```python
from build123d import *

# Parameters (mm, degrees)
F0_R     = 1.27
F0_R_2   = 1.5875
F0_R_3   = 5.55625
F1_DEPTH = 3.175


with BuildPart() as f1:
    # F0 (on Front) → F1 (new body)
    with BuildSketch(Plane.XZ):
        Polygon((4.698286, -12.312303), (38.1, -5.55625), (38.1, 5.55625), (5.55625, 13.26261), (-5.55625, 13.26261), (-38.1, 5.55625), (-38.1, -5.55625), (-4.698286, -12.312303), (-4.698286, -9.621484), (4.698286, -9.621484), align=None)
        with Locations((-6.734358, -6.736026)):
            Circle(F0_R, mode=Mode.SUBTRACT)
        with Locations((-20.32, 0)):
            Circle(F0_R_2, mode=Mode.SUBTRACT)
        with Locations((6.734358, -6.734358)):
            Circle(F0_R, mode=Mode.SUBTRACT)
        Circle(F0_R_3, mode=Mode.SUBTRACT)
        with Locations((20.32, 0)):
            Circle(F0_R_2, mode=Mode.SUBTRACT)
        with Locations((-6.736026, 6.736026)):
            Circle(F0_R, mode=Mode.SUBTRACT)
        with Locations((6.736026, 6.734358)):
            Circle(F0_R, mode=Mode.SUBTRACT)
    extrude(amount=F1_DEPTH)


solid = f1.part
```
Check sheet for the modelled part. Datum: model origin and axes. Units: mm. A direction names the side the tool comes from. Round coordinates to 2 decimals unless told otherwise and drop trailing zeros. Loops run counter-clockwise (first coordinate to the right, second up) from the corner with the lowest first, then second, coordinate; pieces in that order, holes last. Notation, with made-up numbers: (50.25, 40.25) -> (91.25, 40.25) arc R24 ccw to (91.25, 67.25) -> close; hole circle Ø10 at (66.5, -39.5). An arc over 180 degrees is marked (long way). Write item = value, one per line. Start each with the question number.
1) Sectioned sample at C-C, the plane y = -2.2. Record the cut outline in (x, z) (1 decimal), plus the area to 3 significant figures.
2) Set-up check for faces 1 (the flat face through (0, -2, -9.621)), 2 (the flat face through (-1, -3.175, 6)): record each of +Z, -Z, +X, -X, +Y, -Y from which the full face is reachable in a straight line by a thin tool's end or side.
3) Sectioned sample at A-A, the plane x = 0. Record the cut outline in (y, z) (3 decimals), plus the area to 3 significant figures.
4) Thickness scan on probe 1 along Z at (x, y) = (0, -0.9); probe 2 along Z at (x, y) = (-1.5, -2.25); probe 3 along X at (y, z) = (-1.5, 0.5). Record the ranges inside material, lowest first.
5) Sectioned sample at D-D, the plane z = 3.25. Record the cut outline in (x, y) (3 decimals), plus the area to 3 significant figures.
6) Gauge pin test, flat end, axial feed: pin 1 Ø1.9 at (x, z) = (-20.32, 0) entering from +Y. Record the tip position at first contact, or that the pin passes through.
7) Sectioned sample at B-B, the plane z = 0. Record the cut outline in (x, y) (1 decimal).
8) Release check for a two-part mould opening along Z. For faces 3 (the flat face through (-38.1, -2, 0)), 4 (the flat face through (0, -2, 13.263)), 5 (the cylindrical face through (6.569, -1.565, -5.475)) record: released by +Z, released by -Z, zero draft, split by the parting line, or undercut.
Results are:
q1.outline = (-38.1, -5.6) -> (-4.7, -12.3) -> (-4.7, -9.6) -> (4.7, -9.6) -> (4.7, -12.3) -> (38.1, -5.6) -> (38.1, 5.6) -> (5.6, 13.3) -> (-5.6, 13.3) -> (-38.1, 5.6) -> close; hole circle Ø3.2 at (-20.3, 0); hole circle Ø2.5 at (-6.7, -6.7); hole circle Ø2.5 at (-6.7, 6.7); hole circle Ø11.1 at (0, 0); hole circle Ø2.5 at (6.7, -6.7); hole circle Ø2.5 at (6.7, 6.7); hole circle Ø3.2 at (20.3, 0)
q1.area = 1,310 mm^2
q2.face_1 = -Z, +Y, -Y
q2.face_2 = +Z, -Z, +X, -X, -Y
q3.outline = (-3.175, -9.621) -> (0, -9.621) -> (0, -5.556) -> (-3.175, -5.556) -> close; (-3.175, 5.556) -> (0, 5.556) -> (0, 13.263) -> (-3.175, 13.263) -> close
q3.area = 37.4 mm^2
q4.probe_1 = -9.62 to -5.56, 5.56 to 13.26
q4.probe_2 = -9.62 to -5.35, 5.35 to 13.26
q4.probe_3 = -38.1 to -21.83, -18.81 to -5.53, 5.53 to 18.81, 21.83 to 38.1
q5.outline = (-38.1, -3.175) -> (-4.507, -3.175) -> (-4.507, 0) -> (-38.1, 0) -> close; (4.507, -3.175) -> (38.1, -3.175) -> (38.1, 0) -> (4.507, 0) -> close
q5.area = 213 mm^2
q6.pin_1 = through
q7.outline = (-38.1, -3.2) -> (-21.9, -3.2) -> (-21.9, 0) -> (-38.1, 0) -> close; (-18.7, -3.2) -> (-5.6, -3.2) -> (-5.6, 0) -> (-18.7, 0) -> close; (5.6, -3.2) -> (18.7, -3.2) -> (18.7, 0) -> (5.6, 0) -> close; (21.9, -3.2) -> (38.1, -3.2) -> (38.1, 0) -> (21.9, 0) -> close
q8.face_3 = zero draft
q8.face_4 = released by +Z
q8.face_5 = undercut
